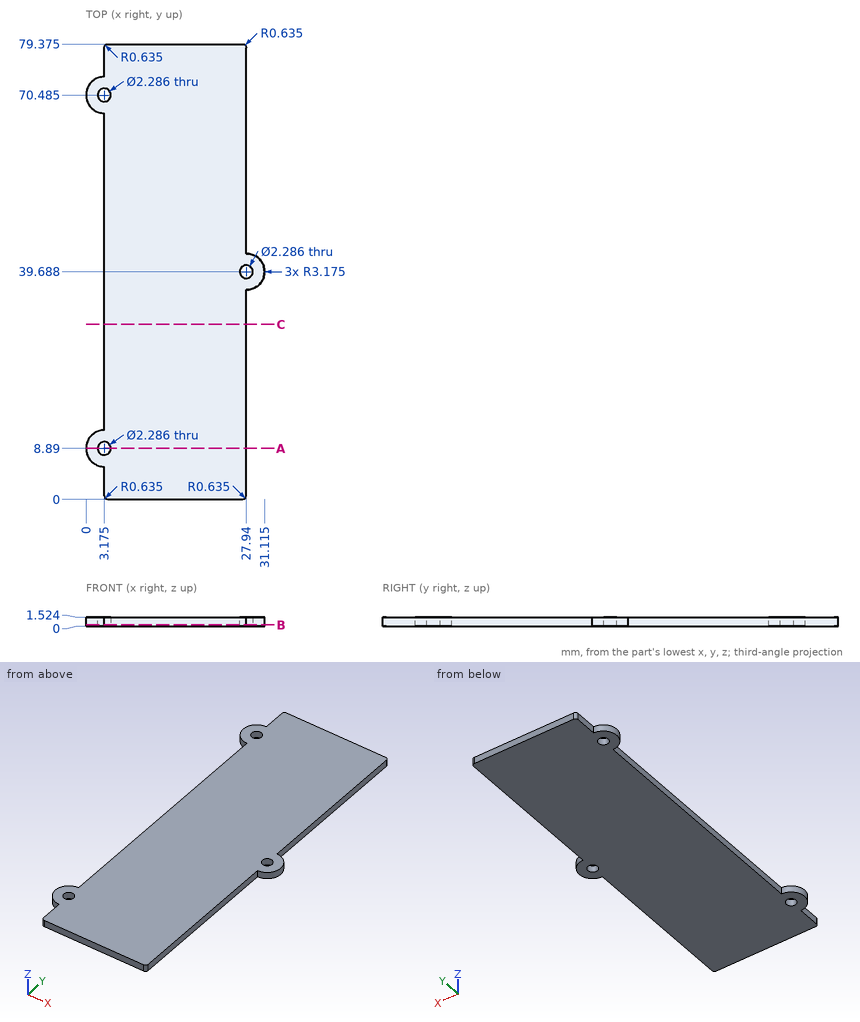
The figure shows three views and two pictorial views of one solid part (mm, origin at its lowest corner). Answer the questions. Give positions to 0.01 mm unless a question says otherwise; leave off trailing zeros. Write each loop counter-clockwise with the first axis right and the second up, starting at its lowest first coordinate (ties: lowest second). Pieces come first, ordered by that corner, then holes. Notation, with made-up numbers: (-35, 21) - (-16, 21) arc R26 ccw to (-16, 41) - close; hole circle Ø5 at (19, -25.75). An arc over 180 degrees is marked (long way). Use CSV: the item, a comma, the result in double quotes. Start each with the question number.
Item 1: The part is cut by section A-A, the plane y = 8.89. Give the vertices of the cut face in (x, z) (1 decimal).
Item 2: Flat-ended cylindrical pins translate along their axes: P1, Ø0.5, axis at y = 62, z = 0.5, coming from the +X side; P2, Ø0.5, axis at y = 4, z = 1, coming from the -X side (1 decimal). Find the tip coordinate at first contact, or state that the pin passes through.
Item 3: The part is cut by section C-C, the plane y = 30.5. Give the vertices of the cut face in (x, z) (1 decimal).
Item 4: The part is cut by section B-B, the plane z = 0.25. Count the separate pieces of the cut face and the enclosed holes in it, and give its area (3 significant figures).
Item 5: Consider line 1 (X direction, y = 66, z = 0.9) (1 decimal); line 2 (Y direction, x = 27, z = 1.3) (1 decimal); line 3 (Y direction, x = 28.5, z = 0.4) (1 decimal). Determine where each line is inside the solid, lowest interval first.
Taken from the geometry:
1,outline,"(0, 0) - (2, 0) - (2, 1.5) - (0, 1.5) - close; (4.3, 0) - (27.9, 0) - (27.9, 1.5) - (4.3, 1.5) - close"
2,P1,"x = 27.94"
2,P2,"x = 3.2"
3,outline,"(3.2, 0) - (27.9, 0) - (27.9, 1.5) - (3.2, 1.5) - close"
4,separate pieces,"1"
4,enclosed holes,"3"
4,area,"2,000 mm2"
5,line 1,"3.2 to 27.9"
5,line 2,"0 to 39, 40.3 to 79.4"
5,line 3,"36.6 to 38.7, 40.7 to 42.8"
